Input: part model. Units: mm. Frame: model coordinates. Face numbers are marked on the shaded views. A direction names the side the tool comes from. Round coordinates to 2 decimals unless told otherwise and drop trailing zeros. Loops run counter-clockwise (first coordinate to the right, second up) from the corner with the lowest first, then second, coordinate; pieces in that order, holes last.
(1) Draft query along X for the marked faces 3, 4 and 5. Return one class per face: released by +X, released by -X, zero draft, split by the parting line, or undercut.
(2) Cut plane D-D, the plane x = 3.25. Output: boundary loops of the cut face in (y, z).
(3) Cut plane A-A, the plane x = 0. Output: boundary loops of the cut face in (y, z).
(4) Line query: line 1 (Z direction, x = 0, y = -2.05); line 2 (Y direction, x = -7.75, z = 7.25); line 3 (X direction, y = -0.5, z = -0.5). Output: solid intervals per line, ascending.
(5) Cut plane B-B, the plane y = -3. Output: boundary loops of the cut face in (x, z).
(6) Cut plane C-C, the plane z = -8.5. Output: boundary loops of the cut face in (x, y), and give its area (3 significant figures).
(7) First-contact query: pin 1 Ø1 at (y, z) = (-3, -6.5) entering from -X; pin 2 Ø4 at (x, z) = (-8, 0) entering from +Y; pin 3 Ø1.5 at (x, y) = (-2.5, 1.5) entering from -Z. Flat tips, straight axial feed; report the tip coordinate or a pass-through.
(8) Access query for the marked faces 1 and 2. Directions: +Z, -Z, +X, -X, +Y, -Y. A direction counts if a zero-diameter tool reaches every point of the face in a straight line with its end or side. Return the directions, or none.
from build123d import *

# Parameters (mm, degrees)
F0_R        = 11
F0_R_2      = 1.75
F0_R_3      = 5.1
F1_DEPTH    = 3.5
F0_R_4      = 4
F2_DEPTH    = 5
F2_FACE_R   = 5.1
F2_FACE_R_2 = 4
F3_DEPTH    = 10


with BuildPart() as f1:
    # F0 (on Front) → F1 (new body)
    with BuildSketch(Plane.XZ):
        Circle(F0_R)
        with Locations((0, -8)):
            Circle(F0_R_2, mode=Mode.SUBTRACT)
        with Locations((-8, 0)):
            Circle(F0_R_2, mode=Mode.SUBTRACT)
        Circle(F0_R_3, mode=Mode.SUBTRACT)
        with Locations((8, 0)):
            Circle(F0_R_2, mode=Mode.SUBTRACT)
        with Locations((0, 8)):
            Circle(F0_R_2, mode=Mode.SUBTRACT)
    extrude(amount=F1_DEPTH)

    # F0 (on Front) → F2 (join)
    with BuildSketch(Plane.XZ):
        Circle(F0_R_3)
        Circle(F0_R_4, mode=Mode.SUBTRACT)
    extrude(amount=F2_DEPTH)

    # F2_face (on face) → F3 (join)
    with BuildSketch(Plane.XZ.offset(5)):
        Circle(F2_FACE_R)
        Circle(F2_FACE_R_2, mode=Mode.SUBTRACT)
    extrude(amount=-F3_DEPTH)


solid = f1.part
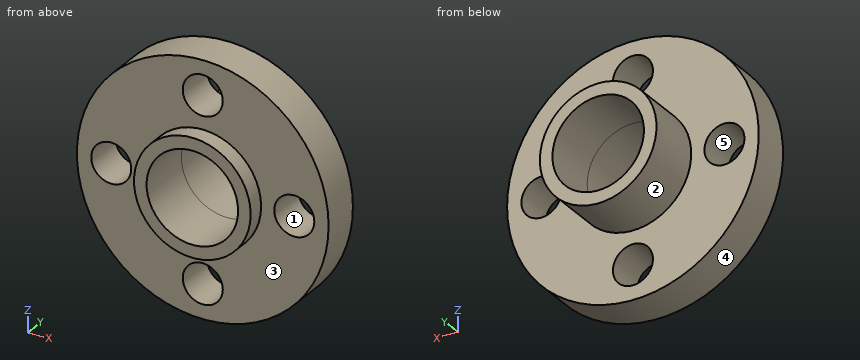
Reported:
1. face 3: zero draft
1. face 4: split by the parting line
1. face 5: undercut
2. outline: (-5, -3.93) - (-3.5, -3.93) - (-3.5, -10.51) - (0, -10.51) - (0, -3.93) - (5, -3.93) - (5, -2.33) - (-5, -2.33) - close; (-5, 2.33) - (5, 2.33) - (5, 3.93) - (0, 3.93) - (0, 10.51) - (-3.5, 10.51) - (-3.5, 3.93) - (-5, 3.93) - close
3. outline: (-5, -5.1) - (-3.5, -5.1) - (-3.5, -6.25) - (0, -6.25) - (0, -5.1) - (5, -5.1) - (5, -4) - (-5, -4) - close; (-5, 4) - (5, 4) - (5, 5.1) - (0, 5.1) - (0, 6.25) - (-3.5, 6.25) - (-3.5, 5.1) - (-5, 5.1) - close; (-3.5, -11) - (0, -11) - (0, -9.75) - (-3.5, -9.75) - close; (-3.5, 9.75) - (0, 9.75) - (0, 11) - (-3.5, 11) - close
4. line 1: z = -11 to -9.75, -6.25 to -4, 4 to 6.25, 9.75 to 11
4. line 2: y = -3.5 to 0
4. line 3: x = -10.99 to -9.68, -6.32 to -3.97, 3.97 to 6.32, 9.68 to 10.99
5. outline: circle Ø22 at (0, 0); hole circle Ø3.5 at (-8, 0); hole circle Ø8 at (0, 0); hole circle Ø3.5 at (0, -8); hole circle Ø3.5 at (0, 8); hole circle Ø3.5 at (8, 0)
6. outline: (-6.98, -3.5) - (-1.68, -3.5) - (-1.68, 0) - (-6.98, 0) - close; (1.68, -3.5) - (6.98, -3.5) - (6.98, 0) - (1.68, 0) - close
6. area: 37.1 mm2
7. pin 1: stops at x = -9.22
7. pin 2: stops at y = 0
7. pin 3: stops at z = -4.79
8. face 1: +Y, -Y
8. face 2: +Y
